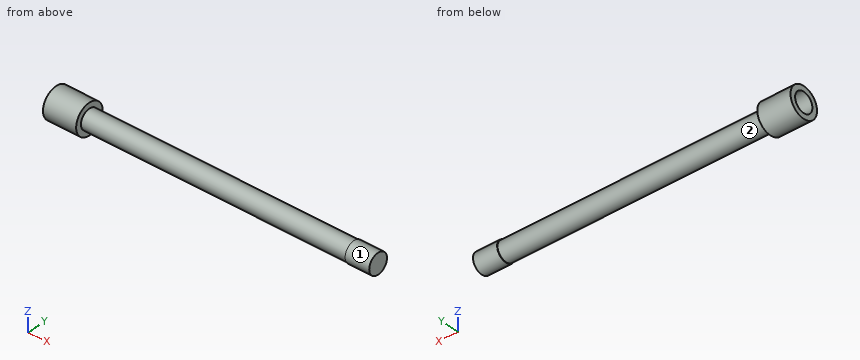
from build123d import *


with BuildPart() as part:
    # Axial profile (mm) → Full revolution (revolve)
    with BuildSketch(Plane.XY, mode=Mode.PRIVATE) as full_revolution_sk:
        Polygon((50, 3.25), (58, 3.25), (58, 0), (156.7, 0), (156.7, 3.35), (148.7, 3.35), (148.7, 3.2), (61, 3.2), (61, 5), (50, 5), align=None)
    revolve(full_revolution_sk.sketch.rotate(Axis((-110, 0, 0), (1, 0, 0)), 90), axis=Axis((-110, 0, 0), (1, 0, 0)))


solid = part.part
Input: part model. Units: mm. Frame: model coordinates. Face numbers are marked on the shaded views. Coordinates: 2 decimals unless noted, no trailing zeros. Write each loop counter-clockwise with the first axis right and the second up, starting at its lowest first coordinate (ties: lowest second). Pieces come first, ordered by that corner, then holes. Notation, with made-up numbers: M 18,31.25 L 64,31.25 A24 ccw 64,58.25 Z; hole C 51,5 d11. An arc over 180 degrees is marked long. Answer as a JSON object with one key per item and string values. Group by question number.
(1) Contact query for flat-ended pins moving along their axis: P1, Ø4, axis at x = 136.5, y = 3.5, coming from the -Z side; P2, Ø6, axis at x = 122.5, z = -3, coming from the +Y side; P3, Ø5, axis at x = 90.5, y = -3, coming from the +Z side. Output: stop coordinate, or through.
(2) Section C-C on x = 67.5. Output: boundary loops of the cut face in (y, z), plus the area to 3 significant figures.
(3) Section A-A on z = 0. Output: boundary loops of the cut face in (x, y), plus the area to 3 significant figures.
(4) Ray query, line 1 along Y through (x, z) = (56.75, 0); line 2 along X through (y, z) = (1, 0.5); line 3 along X through (y, z) = (3.5, 2.5). Return the intervals inside material, ascending. Write a range as [from, to].
(5) Mould query, pull axis X, two halves, no side actions, for the marked faces 1 and 2. Classes: pulls with the +X half, pulls with the -X half, needs draft (parallel to the pull), parting line crosses it, or undercut.
Result set:
{
 "1": {"P1": "stops at z = -2.83", "P2": "stops at y = 3.2", "P3": "stops at z = 3.16"},
 "2": {"outline": "C 0,0 d6.4", "area": "32.2 mm2"},
 "3": {"outline": "M 50,-5 L 61,-5 L 61,-3.2 L 148.7,-3.2 L 148.7,-3.35 L 156.7,-3.35 L 156.7,3.35 L 148.7,3.35 L 148.7,3.2 L 61,3.2 L 61,5 L 50,5 L 50,3.25 L 58,3.25 L 58,-3.25 L 50,-3.25 Z", "area": "673 mm2"},
 "4": {"line 1": "y = [-5, -3.25], [3.25, 5]", "line 2": "x = [58, 156.7]", "line 3": "x = [50, 61]"},
 "5": {"face 1": "needs draft", "face 2": "undercut"}
}
